Check sheet for the modelled part. Datum: model origin and axes. Units: mm. Face numbers are marked on the shaded views. A direction names the side the tool comes from. Round coordinates to 2 decimals unless told otherwise and drop trailing zeros. Order: outer loops, then holes, each group sorted by start corner. A loop starts at its lowest first (then second) coordinate and runs counter-clockwise, first axis right, second up. Notation, with made-up numbers: (64.25, -36) -> (119.25, -36) arc R15 ccw to (119.25, -15) -> close; hole circle Ø10 at (20.5, 50). An arc over 180 degrees is marked (long way). Answer in a Markdown table with one row per item.
from build123d import *

# Parameters (mm, degrees)
F1_DEPTH = 15
F2_R     = 18.75
F3_DEPTH = 40


# Not quite as in the source:
# - a fillet or chamfer that OpenCascade refuses, or shapes differently, is made with other operations: its cross-section is extruded or revolved along the edge and cut away or added


with BuildPart() as f1:
    # F0 (on Front) → F1 (new body)
    with BuildSketch(Plane.XZ):
        Polygon((-15, 40.5656324383), (-35, 40.5656324383), (-30, 25.5656324383), (-15, 25.5656324383), align=None)
        Polygon((5, 40.5656324383), (-15, 40.5656324383), (-15, 25.5656324383), (0, 25.5656324383), align=None)
        Polygon((-15, 25.5656324383), (-30, 25.5656324383), (-45, 25.5656324383), (-30, -19.4343675617), (0, -19.4343675617), (15, 25.5656324383), (0, 25.5656324383), align=None)
    extrude(amount=F1_DEPTH)

    # F2 (on face) → F3 (join)
    with BuildSketch(Plane(origin=(0, 0, -19.4343675617), x_dir=(1, 0, 0), z_dir=(0, 0, -1))):
        with Locations((-15, 7.5)):
            Circle(F2_R)
    extrude(amount=F3_DEPTH)

    # F4: chamfer of 10 x 40 on 1 edges, made by hand


with BuildPart() as f4_tool2:
    # F4_s3 → F4_t4 (revolve)
    with BuildSketch(Plane.XZ.offset(7.5)):
        Polygon((3.75, -59.4343675617), (-6.25, -19.4343675617), (3.75, -19.4343675617), align=None)
    revolve(axis=Axis((-15, -7.5, -19.4343675617), (0, 0, -1)))

    split(bisect_by=Plane(origin=(5.8303102685, 0, -1.9434367562), x_dir=(0, 1, 0), z_dir=(0.9486832981, 0, -0.316227766)), keep=Keep.TOP)


with BuildPart() as f1_1:
    add(f1.part)

    # F4_t1: cut F4_tool2
    add(f4_tool2.part, mode=Mode.SUBTRACT)


with BuildPart() as f4_tool7:
    # F4_s8 → F4_t9 (revolve)
    with BuildSketch(Plane.XZ.offset(7.5)):
        Polygon((3.75, -59.4343675617), (-6.25, -19.4343675617), (3.75, -19.4343675617), align=None)
    revolve(axis=Axis((-15, -7.5, -19.4343675617), (0, 0, -1)))

    split(bisect_by=Plane.XZ.offset(15), keep=Keep.TOP)


with BuildPart() as f1_2:
    add(f1_1.part)

    # F4_t6: cut F4_tool7
    add(f4_tool7.part, mode=Mode.SUBTRACT)


with BuildPart() as f4_tool12:
    # F4_s13 → F4_t14 (revolve)
    with BuildSketch(Plane.XZ.offset(7.5)):
        Polygon((3.75, -59.4343675617), (-6.25, -19.4343675617), (3.75, -19.4343675617), align=None)
    revolve(axis=Axis((-15, -7.5, -19.4343675617), (0, 0, -1)))

    split(bisect_by=Plane.XZ, keep=Keep.BOTTOM)


with BuildPart() as f1_3:
    add(f1_2.part)

    # F4_t11: cut F4_tool12
    add(f4_tool12.part, mode=Mode.SUBTRACT)


with BuildPart() as f4_tool17:
    # F4_s18 → F4_t19 (revolve)
    with BuildSketch(Plane.XZ.offset(7.5)):
        Polygon((3.75, -59.4343675617), (-6.25, -19.4343675617), (3.75, -19.4343675617), align=None)
    revolve(axis=Axis((-15, -7.5, -19.4343675617), (0, 0, -1)))

    split(bisect_by=Plane(origin=(-32.8303102685, 0, -10.9434367562), x_dir=(0, 1, 0), z_dir=(-0.9486832981, 0, -0.316227766)), keep=Keep.TOP)


with BuildPart() as f1_4:
    add(f1_3.part)

    # F4_t16: cut F4_tool17
    add(f4_tool17.part, mode=Mode.SUBTRACT)


solid = f1_4.part
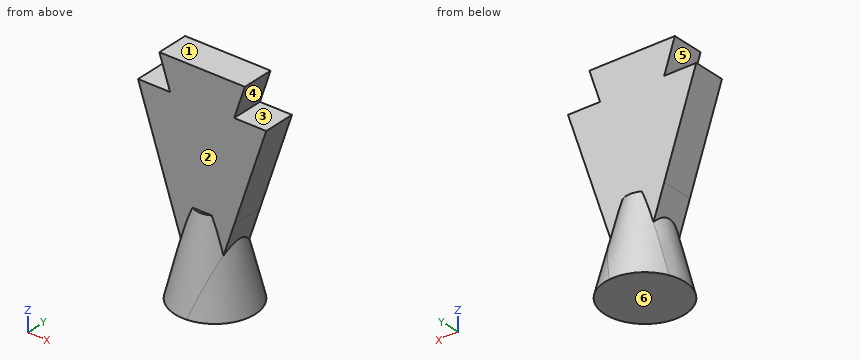
Item 1: Mould release check, pull along Z, two halves, no side actions. Record for the marked faces 1, 2 and 3: pulls with the +Z half, pulls with the -Z half, needs draft (parallel to the pull), parting line crosses it, or undercut.
Result sheet:
| item | result |
|---|---|
| face 1 | pulls with the +Z half |
| face 2 | needs draft |
| face 3 | undercut |
Item 2: Cross-section at A-A (z = -25). Record the boundary of the cut face in (x, y).
Result sheet:
| item | result |
|---|---|
| outline | (-28.14, -15) -> (-21.83, -15) arc R10.14 ccw to (-8.17, -15) -> (-1.86, -15) -> (-1.86, 0) -> (-8.17, 0) arc R10.14 ccw to (-21.83, 0) -> (-28.14, 0) -> close |
Item 3: Cross-section at B-B (x = 10). Record the boundary of the cut face in (y, z), and give its area (3 significant figures).
Result sheet:
| item | result |
|---|---|
| outline | (-15, 10.57) -> (0, 10.57) -> (0, 25.57) -> (-15, 25.57) -> close |
| area | 225 mm^2 |
Item 4: Set-up check for the marked faces 4, 5 and 6: record each of +Z, -Z, +X, -X, +Y, -Y from which the full face is reachable in a straight line by a thin tool's end or side.
Result sheet:
| item | result |
|---|---|
| face 4 | +X, +Y, -Y |
| face 5 | -X, +Y, -Y |
| face 6 | -Z, +X, -X, +Y, -Y |
Item 5: Depth check by flat-ended pin: P1, Ø10, axis at x = -22.5, z = -25, coming from the +Y side; P2, Ø1, axis at x = -17, z = -39, coming from the +Y side; P3, Ø1, axis at y = -12, z = 8, coming from the -X side; P4, Ø6, axis at y = 5, z = 9.5, coming from the +X side. Enter the tip coordinate at first touch or a pass-through.
Result sheet:
| item | result |
|---|---|
| P1 | stops at y = 2.81 |
| P2 | stops at y = 6.14 |
| P3 | stops at x = -39.31 |
| P4 | passes through |
Item 6: Scan lines: line 1 (Y direction, x = -9.5, z = 0); line 2 (X direction, y = 1.5, z = -37); line 3 (X direction, y = -8, z = 2.5). Record each from-to range of solid material in increasing order. Write a range as [from, to].
Result sheet:
| item | result |
|---|---|
| line 1 | y = [-15, 0] |
| line 2 | x = [-24.58, -5.42] |
| line 3 | x = [-37.31, 7.31] |
Item 7: Cross-section at D-D (z = -40). Record the boundary of the cut face in (x, y).
Result sheet:
| item | result |
|---|---|
| outline | circle Ø27.78 at (-15, -7.5) |
Item 8: Cross-section at C-C (z = -3.5). Record the boundary of the cut face in (x, y).
Result sheet:
| item | result |
|---|---|
| outline | (-35.31, -15) -> (5.31, -15) -> (5.31, 0) -> (-35.31, 0) -> close |
